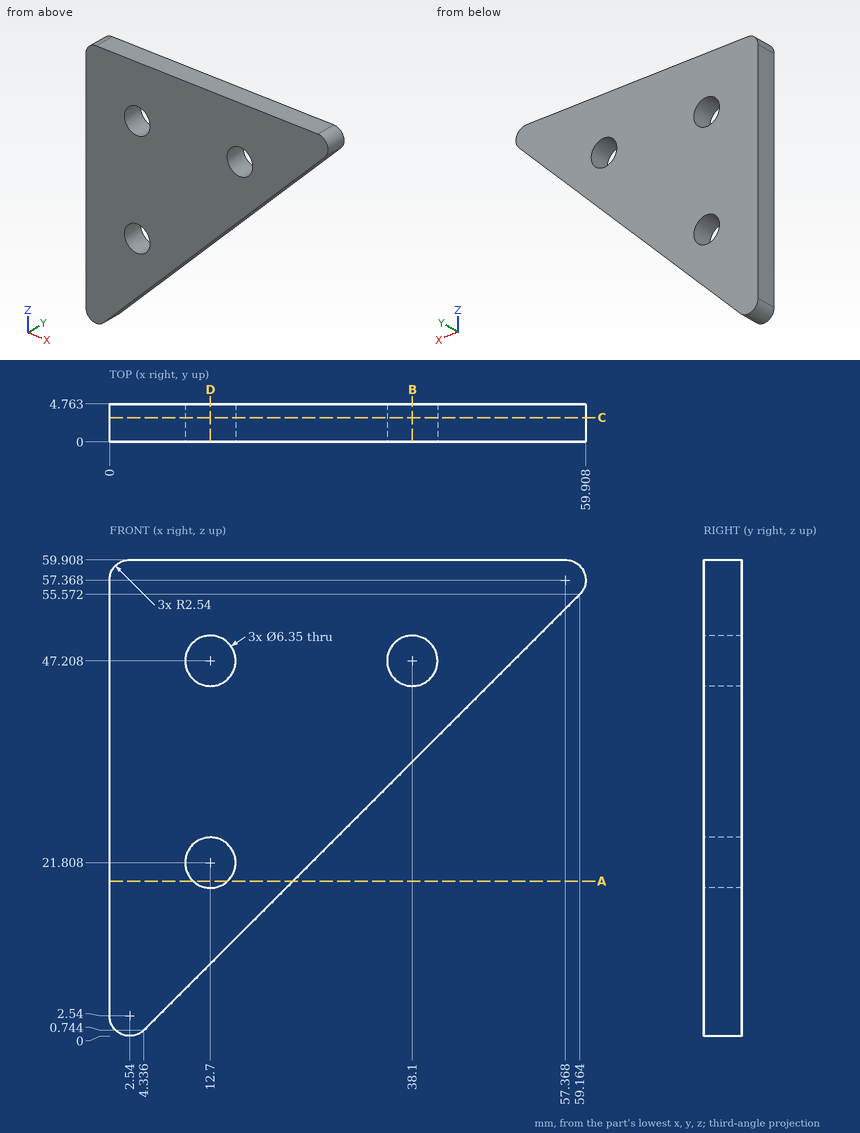
Geometry: see drawing. Coordinates: mm, zero at the bounding-box minimum. Coordinates: 2 decimals unless noted, no trailing zeros. Loops run counter-clockwise (first coordinate to the right, second up) from the corner with the lowest first, then second, coordinate; pieces in that order, holes last. Notation, with made-up numbers: (42, 15.5) - (100, 15.5) arc R21 cw to (100, 22.5) - close; hole circle Ø6 at (76.25, 23.25). An arc over 180 degrees is marked (long way). Return JSON: item names as keys, results as strings.
Q1. Section C-C, the plane y = 3.05. Give the number of separate pieces and of enclosed holes in the cut face, plus the area to 3 significant figures.
Results:
{"separate pieces": "1", "enclosed holes": "3", "area": "1,900 mm2"}
Q2. Section D-D, the plane x = 12.7. Return loops of the section in (y, z).
Results:
{"outline": "(0, 9.11) - (4.76, 9.11) - (4.76, 18.63) - (0, 18.63) - close; (0, 24.98) - (4.76, 24.98) - (4.76, 44.03) - (0, 44.03) - close; (0, 50.38) - (4.76, 50.38) - (4.76, 59.91) - (0, 59.91) - close"}
Q3. Section B-B, the plane x = 38.1. Return loops of the section in (y, z).
Results:
{"outline": "(0, 34.51) - (4.76, 34.51) - (4.76, 44.03) - (0, 44.03) - close; (0, 50.38) - (4.76, 50.38) - (4.76, 59.91) - (0, 59.91) - close"}
Q4. Material intervals for line 1 along X through (y, z) = (2.6, 44.5) (1 decimal); line 2 along Z through (x, y) = (15.5, 2.3) (1 decimal); line 3 along Z through (x, y) = (41, 0.9) (1 decimal), sorted ascending.
Results:
{"line 1": "0 to 11, 14.4 to 36.4, 39.8 to 48.1", "line 2": "11.9 to 20.3, 23.3 to 45.7, 48.7 to 59.9", "line 3": "37.4 to 45.9, 48.5 to 59.9"}
Q5. Section A-A, the plane z = 19.5. Return loops of the section in (x, y).
Results:
{"outline": "(0, 0) - (10.52, 0) - (10.52, 4.76) - (0, 4.76) - close; (14.88, 0) - (23.09, 0) - (23.09, 4.76) - (14.88, 4.76) - close"}
Q6. Contact query for flat-ended pins moving along their axis: P1, Ø2, axis at x = 6.5, y = 1, coming from the -Z side; P2, Ø1, axis at x = 48, y = 2, coming from the -Z side. Output: stop coordinate, or through.
Results:
{"P1": "z = 1.91", "P2": "z = 43.91"}
